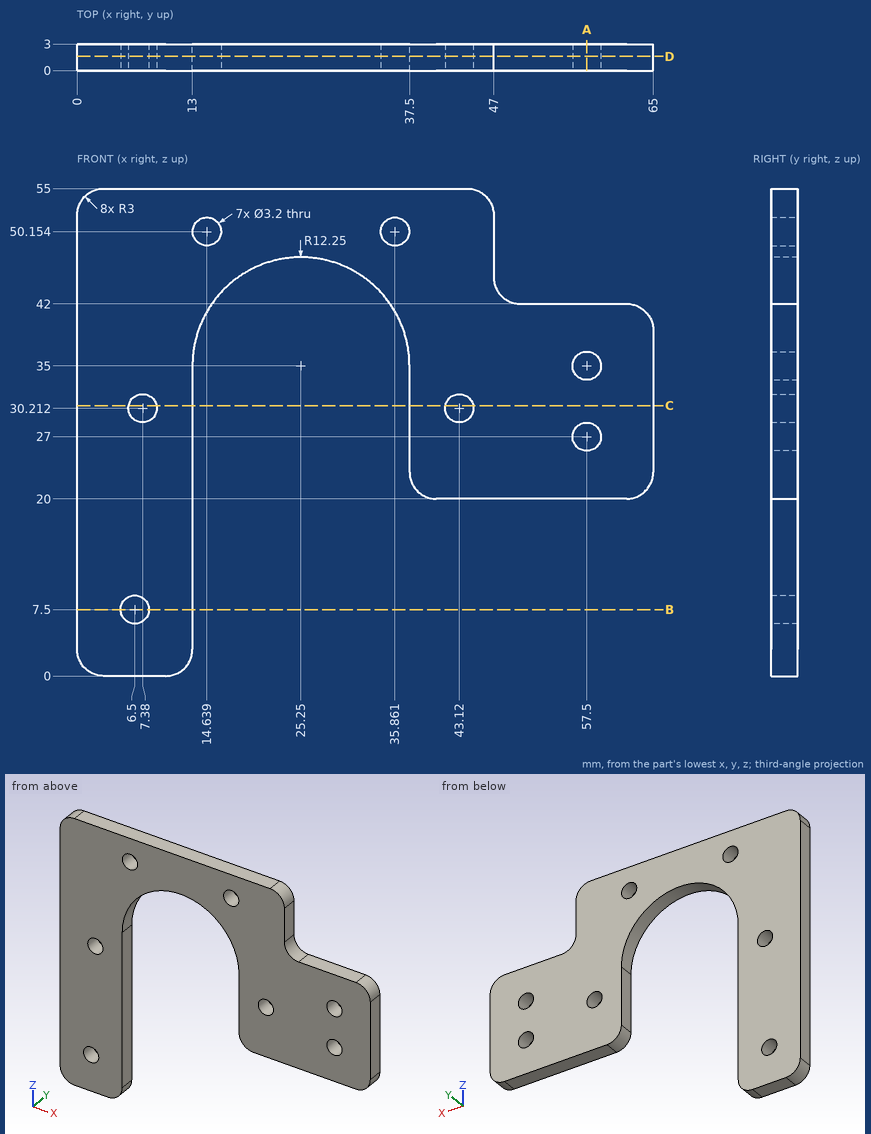
Geometry: see drawing. Coordinates: mm, zero at the bounding-box minimum. Coordinates: 2 decimals unless noted, no trailing zeros. Loops run counter-clockwise (first coordinate to the right, second up) from the corner with the lowest first, then second, coordinate; pieces in that order, holes last. Notation, with made-up numbers: (73, 13) -> (90, 13) arc R15 ccw to (90, 40) -> close; hole circle Ø9 at (-14.75, -30.5). An arc over 180 degrees is marked (long way). Write item = value, one per line. Start each with the question number.
Item 1: Cut plane D-D, the plane y = 1.6. Count the separate pieces of the cut face and the enclosed holes in it, plus the area to 3 significant figures.
Item 2: Cut plane A-A, the plane x = 57.5. Return loops of the section in (y, z), plus the area to 3 significant figures.
Item 3: Cut plane C-C, the plane z = 30.5. Return loops of the section in (x, y), plus the area to 3 significant figures.
Item 4: Cut plane B-B, the plane z = 7.5. Return loops of the section in (x, y), plus the area to 3 significant figures.
Item 5: First-contact query: P1, Ø2.5, axis at x = 35.86, z = 50.15, coming from the -Y side; P2, Ø1.5, axis at x = 58, y = 1.5, coming from the +Z side. Flat tips, straight axial feed; report the tip coordinate or a pass-through.
Item 6: Material intervals for line 1 (X direction, y = 1.35, z = 27); line 2 (X direction, y = 2.25, z = 31); line 3 (X direction, y = 1.65, z = 12), sorted ascending.
Ans:
q1.separate_pieces = 1
q1.enclosed_holes = 7
q1.area = 1,630 mm²
q2.outline = (0, 20) -> (3, 20) -> (3, 25.4) -> (0, 25.4) -> close; (0, 28.6) -> (3, 28.6) -> (3, 33.4) -> (0, 33.4) -> close; (0, 36.6) -> (3, 36.6) -> (3, 42) -> (0, 42) -> close
q2.area = 46.8 mm²
q3.outline = (0, 0) -> (5.81, 0) -> (5.81, 3) -> (0, 3) -> close; (8.95, 0) -> (13, 0) -> (13, 3) -> (8.95, 3) -> close; (37.5, 0) -> (41.55, 0) -> (41.55, 3) -> (37.5, 3) -> close; (44.69, 0) -> (65, 0) -> (65, 3) -> (44.69, 3) -> close
q3.area = 103 mm²
q4.outline = (0, 0) -> (4.9, 0) -> (4.9, 3) -> (0, 3) -> close; (8.1, 0) -> (13, 0) -> (13, 3) -> (8.1, 3) -> close
q4.area = 29.4 mm²
q5.P1 = through
q5.P2 = 42
q6.line_1 = 0 to 13, 37.5 to 55.9, 59.1 to 65
q6.line_2 = 0 to 5.99, 8.77 to 13, 37.5 to 41.73, 44.51 to 65
q6.line_3 = 0 to 13
